Design review of the part shown in the three views and the two pictorial views. Dimensions are in mm from the part's minimum x, y and z. A direction names the side the tool comes from. Round coordinates to 2 decimals unless told otherwise and drop trailing zeros. Loops run counter-clockwise (first coordinate to the right, second up) from the corner with the lowest first, then second, coordinate; pieces in that order, holes last. Notation, with made-up numbers: M 4,14 L 62,14 A23 ccw 62,43 Z; hole C 1,30.5 d1. An arc over 180 degrees is marked long. One line per question, with ' | ' between items. Start each with the question number.
1) We need section C-C (z = 34). Give the boundary of the cut face in (x, y).
2) For the marked faces 1, 2, 3 and 4, list the 3-axis set-ups (+Z, -Z, +X, -X, +Y, -Y) from which the entire face can be reached by the end or side of a thin tool; tool diameter is ignored.
3) Mouldability with a two-part tool opening along X and no side actions: class the marked faces 5, 6, 7 and 8 as pulls with the +X half, pulls with the -X half, needs draft (parallel to the pull), parting line crosses it, or undercut.
4) We need section B-B (y = 20). Give the boundary of the cut face in (x, z).
5) For pin 1 Ø6 at (y, z) = (20, 15) entering from +X; pin 2 Ø12 at (x, y) = (23, 30) entering from -Z; pin 3 Ø5 at (x, z) = (9, 24) entering from +Y; pin 4 Ø5 at (x, z) = (4.5, 23.5) entering from -Y, all flat-tipped, find the tip position at first contact; note any pin that passes through.
6) For probe 1 along Z at (x, y) = (52, 20); probe 2 along X at (y, z) = (13.5, 8.5); probe 3 along Y at (x, z) = (3.5, 12), list the stretches that pass through material, from the lowest coordinate up. Write a range as from..to.
7) We need section A-A (x = 30). Give the boundary of the cut face in (y, z), and give its area (3 significant figures).
8) We need section D-D (y = 27). Give the boundary of the cut face in (x, z), and give its area (3 significant figures).
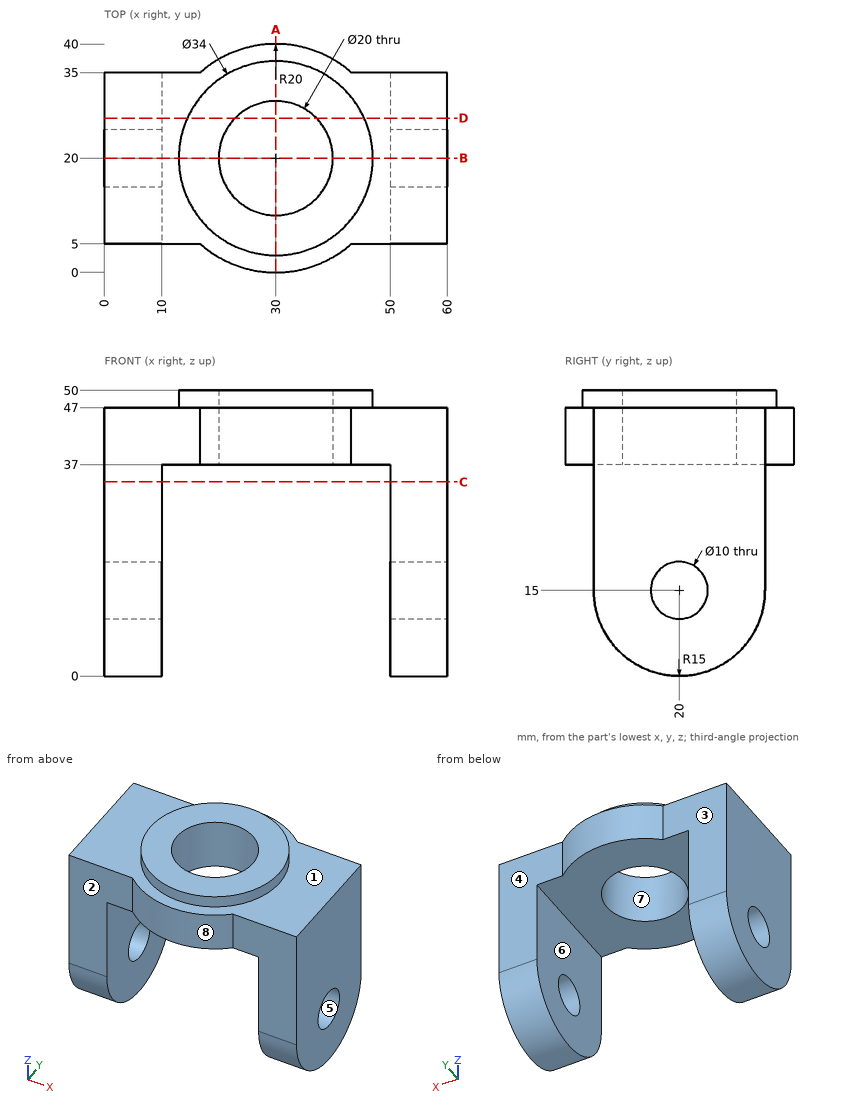
Answers below:
1) outline: M 0,5 L 10,5 L 10,35 L 0,35 Z; M 50,5 L 60,5 L 60,35 L 50,35 Z
2) face 1: +Z | face 2: +Z, -Z, -X, -Y | face 3: +Z, -Z, -X, +Y | face 4: +Z, -Z, +X, +Y
3) face 5: needs draft | face 6: undercut | face 7: undercut | face 8: parting line crosses it
4) outline: M 0,0 L 10,0 L 10,10 L 0,10 Z; M 0,20 L 10,20 L 10,37 L 20,37 L 20,50 L 13,50 L 13,47 L 0,47 Z; M 40,37 L 50,37 L 50,20 L 60,20 L 60,47 L 47,47 L 47,50 L 40,50 Z; M 50,0 L 60,0 L 60,10 L 50,10 Z
5) pin 1: through | pin 2: z = 37 | pin 3: y = 35 | pin 4: y = 5
6) probe 1: 0..10, 20..47 | probe 2: 0..10, 50..60 | probe 3: 5.3..16, 24..34.7
7) outline: M 0,37 L 10,37 L 10,50 L 3,50 L 3,47 L 0,47 Z; M 30,37 L 40,37 L 40,47 L 37,47 L 37,50 L 30,50 Z | area: 242 mm^2
8) outline: M 0,1.73 L 10,1.73 L 10,37 L 22.86,37 L 22.86,50 L 14.51,50 L 14.51,47 L 0,47 Z; M 37.14,37 L 50,37 L 50,1.73 L 60,1.73 L 60,47 L 45.49,47 L 45.49,50 L 37.14,50 Z | area: 1,210 mm^2
